from build123d import *

# Parameters (mm, degrees)
SKETCH1_R      = 4.25
SKETCH1_R_2    = 1.65
SKETCH1_R_3    = 11.25
SKETCH1_W      = 5
SKETCH1_H      = 20.5
EXTRUDE1_DEPTH = 8
SKETCH2_R      = 1
EXTRUDE2_DEPTH = 1
SKETCH3_R      = 1.75
EXTRUDE3_DEPTH = 10


with BuildPart() as part:
    # Sketch1 → Extrude1 (new body)
    with BuildSketch(Plane(origin=(0, 0, 0), x_dir=(1, 0, 0), z_dir=(0, 1, 0))):
        with BuildLine():
            Line((4.894189333, 14.494689664), (4.894189333, 89.494689664))
            ThreePointArc((4.894189333, 89.494689664), (6.651548646, 93.737330351), (10.894189333, 95.494689664))
            Line((10.894189333, 95.494689664), (61.894189333, 95.494689664))
            ThreePointArc((61.894189333, 95.494689664), (66.136830021, 93.737330351), (67.894189333, 89.494689664))
            Line((67.894189333, 89.494689664), (67.894189333, 14.494689664))
            Line((67.894189333, 14.494689664), (66.894189333, 13.494689664))
            Line((66.894189333, 13.494689664), (52.894189333, 13.494689664))
            Line((52.894189333, 13.494689664), (52.894189333, 5.994689664))
            Line((52.894189333, 5.994689664), (51.894189333, 4.994689664))
            Line((51.894189333, 4.994689664), (45.394189333, 4.994689664))
            Line((45.394189333, 4.994689664), (44.394189333, 5.994689664))
            Line((44.394189333, 5.994689664), (44.394189333, 13.494689664))
            Line((44.394189333, 13.494689664), (38.144189333, 13.494689664))
            Line((38.144189333, 13.494689664), (38.144189333, 17.994689664))
            Line((38.144189333, 17.994689664), (39.144189333, 17.994689664))
            Line((39.144189333, 17.994689664), (39.144189333, 20.494689664))
            Line((39.144189333, 20.494689664), (38.144189333, 20.494689664))
            Line((38.144189333, 20.494689664), (38.144189333, 25.494689664))
            Line((38.144189333, 25.494689664), (34.644189333, 25.494689664))
            Line((34.644189333, 25.494689664), (34.644189333, 20.494689664))
            Line((34.644189333, 20.494689664), (33.644189333, 20.494689664))
            Line((33.644189333, 20.494689664), (33.644189333, 17.994689664))
            Line((33.644189333, 17.994689664), (34.644189333, 17.994689664))
            Line((34.644189333, 17.994689664), (34.644189333, 13.494689664))
            Line((34.644189333, 13.494689664), (28.394189333, 13.494689664))
            Line((28.394189333, 13.494689664), (28.394189333, 5.994689664))
            Line((28.394189333, 5.994689664), (27.394189333, 4.994689664))
            Line((27.394189333, 4.994689664), (20.894189333, 4.994689664))
            Line((20.894189333, 4.994689664), (19.894189333, 5.994689664))
            Line((19.894189333, 5.994689664), (19.894189333, 13.494689664))
            Line((19.894189333, 13.494689664), (5.894189333, 13.494689664))
            Line((5.894189333, 13.494689664), (4.894189333, 14.494689664))
        make_face()
        with Locations(Location((13.394189333, 72.994689664, 0), (0, 0, 270))):
            Circle(SKETCH1_R, mode=Mode.SUBTRACT)
        with Locations(Location((51.894189333, 88.494689664, 0), (0, 0, 270))):
            Circle(SKETCH1_R_2, mode=Mode.SUBTRACT)
        with Locations(Location((20.894189333, 88.494689664, 0), (0, 0, 270))):
            Circle(SKETCH1_R_2, mode=Mode.SUBTRACT)
        with Locations(Location((51.894189333, 57.494689664, 0), (0, 0, 270))):
            Circle(SKETCH1_R_2, mode=Mode.SUBTRACT)
        with Locations(Location((20.894189333, 57.494689664, 0), (0, 0, 270))):
            Circle(SKETCH1_R_2, mode=Mode.SUBTRACT)
        with Locations(Location((36.394189333, 72.994689664, 0), (0, 0, 270))):
            Circle(SKETCH1_R_3, mode=Mode.SUBTRACT)
        with Locations((9.394189333, 54.494689664)):
            Rectangle(SKETCH1_W, SKETCH1_H, mode=Mode.SUBTRACT)
        with Locations((63.394189333, 54.494689664)):
            Rectangle(SKETCH1_W, SKETCH1_H, mode=Mode.SUBTRACT)
    extrude(amount=EXTRUDE1_DEPTH)

    # Sketch2 → Extrude2 (cut)
    with BuildSketch(Plane.XY.offset(-25.494689664)):
        with Locations((36.394189333, 4)):
            Circle(SKETCH2_R)
    extrude(amount=-EXTRUDE2_DEPTH, mode=Mode.SUBTRACT)

    # Sketch3 → Extrude3 (cut)
    with BuildSketch(Plane(origin=(0, 8, 0), x_dir=(1, 0, 0), z_dir=(0, 1, 0))):
        with Locations(Location((9.394189333, 82.994689664, 0), (0, 0, 270))):
            Circle(SKETCH3_R)
        with Locations(Location((63.394189333, 82.994689664, 0), (0, 0, 270))):
            Circle(SKETCH3_R)
    extrude(amount=-EXTRUDE3_DEPTH, mode=Mode.SUBTRACT)


solid = part.part
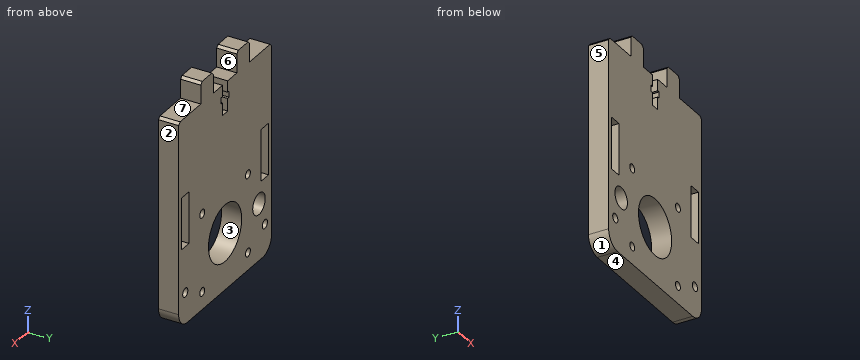
Source: CAD feature listing. Evaluate the final solid. Frame: model axes, mm. Face numbers are marked on the shaded views. A direction names the side the tool comes from. Coordinates: 2 decimals unless noted, no trailing zeros. Order: outer loops, then holes, each group sorted by start corner. A loop starts at its lowest first (then second) coordinate and runs counter-clockwise, first axis right, second up.
Item 1: Material intervals for line 1 (X direction, y = 3.25, z = -55.5); line 2 (Z direction, x = 63, y = 0.75); line 3 (X direction, y = 4.75, z = -56.5), sorted ascending.
Output values:
line 1: x = 4.89 to 6.89, 11.89 to 60.89, 65.89 to 67.89
line 2: z = -95.39 to -84.7, -81.29 to -64.74, -44.24 to -13.49
line 3: x = 4.89 to 6.89, 11.89 to 19.58, 22.21 to 50.58, 53.21 to 60.89, 65.89 to 67.89
Item 2: Cut plane C-C (y = 4). Count the separate pieces of the cut face and the enclosed holes in it, plus the area to 3 significant figures.
Output values:
separate pieces: 1
enclosed holes: 10
area: 4,530 mm2
Item 3: First-contact query: P1, Ø1.5, axis at x = 62.5, y = 2, coming from the +Z side; P2, Ø1, axis at x = 37, y = 3.5, coming from the +Z side; P3, Ø5.5, axis at x = 20.89, z = -88.49, coming from the -Y side; P4, Ø2.5, axis at x = 8.5, y = 6, coming from the -Z side. Flat tips, straight axial feed; report the tip coordinate or a pass-through.
Output values:
P1: stops at z = -13.49
P2: stops at z = -25.49
P3: stops at y = 0
P4: stops at z = -95.38
Item 4: Cut plane A-A (z = -49.5). Return loops of the section in (x, y).
Output values:
outline: (4.89, 0) - (6.89, 0) - (6.89, 8) - (4.89, 8) - close; (11.89, 0) - (60.89, 0) - (60.89, 8) - (11.89, 8) - close; (65.89, 0) - (67.89, 0) - (67.89, 8) - (65.89, 8) - close
Item 5: Cut plane D-D (x = 57). Return loops of the section in (y, z), plus the area to 3 significant figures.
Output values:
outline: (0, -95.49) - (8, -95.49) - (8, -13.49) - (0, -13.49) - close
area: 656 mm2
Item 6: Cut plane B-B (x = 15). Return loops of the section in (y, z), plus the area to 3 significant figures.
Output values:
outline: (0, -95.49) - (8, -95.49) - (8, -76.93) - (0, -76.93) - close; (0, -69.06) - (8, -69.06) - (8, -13.49) - (0, -13.49) - close
area: 593 mm2
Item 7: Pull-direction query (X, two-part tool) for the marked faces 1, 2, 3 and 4; classes: pulls with the +X half, pulls with the -X half, needs draft (parallel to the pull), parting line crosses it, or undercut.
Output values:
face 1: pulls with the -X half
face 2: pulls with the +X half
face 3: undercut
face 4: needs draft
Item 8: Set-up query: the marked faces 5, 6 and 7. Return all of +Z, -Z, +X, -X, +Y, -Y with unobstructed straight access to the full face (end or side cutting, diameter ignored); none if empty.
Output values:
face 5: +Z, -Z, -X, +Y, -Y
face 6: +Z, +Y, -Y
face 7: +Z, +X, +Y, -Y
